The figure shows three views and two pictorial views of one solid part (mm, origin at its lowest corner). Answer the questions. Coordinates: 2 decimals unless noted, no trailing zeros. Write each loop counter-clockwise with the first axis right and the second up, starting at its lowest first coordinate (ties: lowest second). Pieces come first, ordered by that corner, then holes. Notation, with made-up numbers: M -36,-34.75 L 3,-34.75 A21 cw 3,4.25 Z; hole C 57.5,11.25 d1. An arc over 180 degrees is marked long. Answer as CSV lines item,"result".
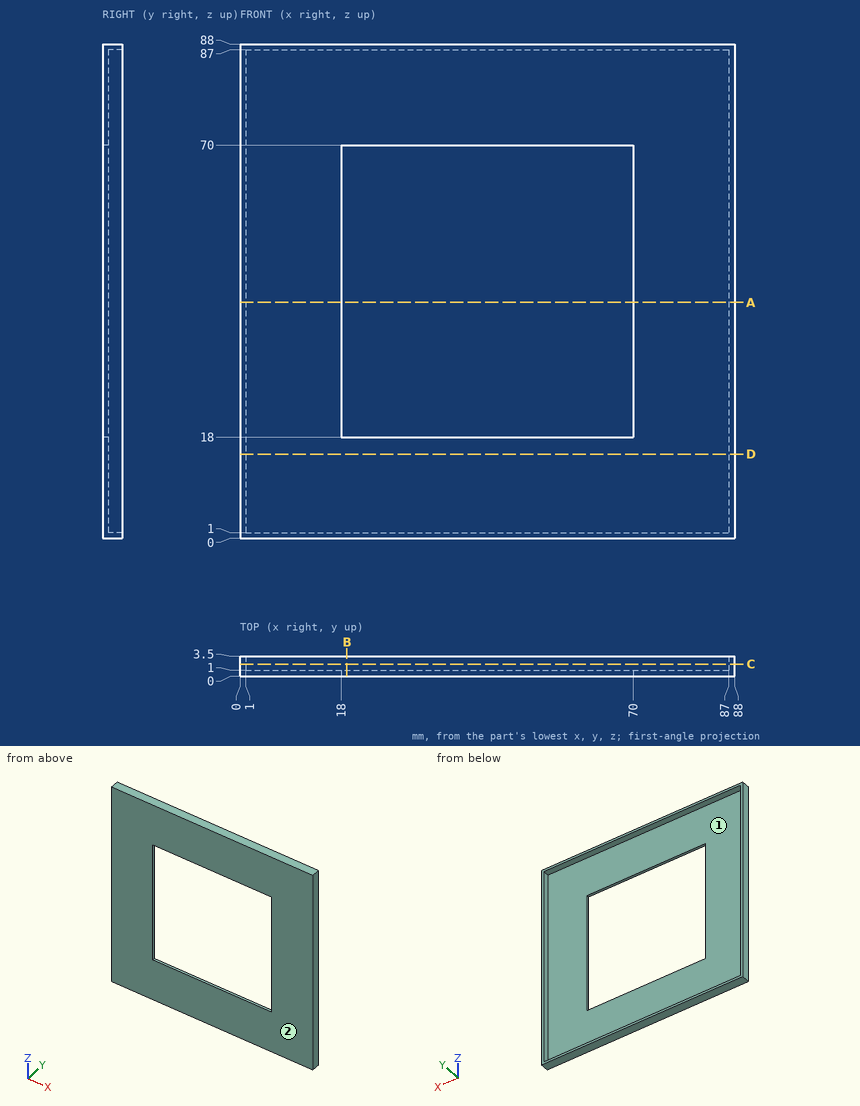
Q1. Find section D-D (z = 15). Give the vertices of the cut face in (x, y).
Output:
outline,"M 0,0 L 88,0 L 88,3.5 L 87,3.5 L 87,1 L 1,1 L 1,3.5 L 0,3.5 Z"
Q2. Find section A-A (z = 42). Give the vertices of the cut face in (x, y), and give its area (3 significant figures).
Output:
outline,"M 0,0 L 18,0 L 18,1 L 1,1 L 1,3.5 L 0,3.5 Z; M 70,0 L 88,0 L 88,3.5 L 87,3.5 L 87,1 L 70,1 Z"
area,"41.0 mm2"
Q3. The mould has two halves that part along Z. Classify the marked faces 1 and 2: pulls with the +Z half, pulls with the -Z half, needs draft (parallel to the pull), parting line crosses it, or undercut.
Output:
face 1,"undercut"
face 2,"needs draft"
Q4. Flat-ended cylindrical pins translate along their axes: pin 1 Ø1.5 at (x, z) = (25, 20.5) entering from +Y; pin 2 Ø4 at (x, z) = (9, 43.5) entering from -Y; pin 3 Ø8 at (x, z) = (59.5, 18.5) entering from +Y. Find the tip coordinate at first contact, or state that the pin passes through.
Output:
pin 1,"through"
pin 2,"y = 0"
pin 3,"y = 1"
Q5. Find section B-B (x = 19). Give the vertices of the cut face in (y, z), and give its area (3 significant figures).
Output:
outline,"M 0,0 L 3.5,0 L 3.5,1 L 1,1 L 1,18 L 0,18 Z; M 0,70 L 1,70 L 1,87 L 3.5,87 L 3.5,88 L 0,88 Z"
area,"41.0 mm2"
Q6. Straight lines are drawn through the part: line 1 (Z direction, x = 40, y = 0.6); line 2 (X direction, y = 2.5, z = 6). For each, find the intervals that lie inside material, in ascending order.
Output:
line 1,"0 to 18, 70 to 88"
line 2,"0 to 1, 87 to 88"
Q7. Find section C-C (y = 2.1). Give the vertices of the cut face in (x, z).
Output:
outline,"M 0,0 L 88,0 L 88,88 L 0,88 Z; hole M 1,1 L 87,1 L 87,87 L 1,87 Z"
